Solid Edge part; units mm, degrees
sketch "Sketch1" plane through (0, 0, 0) normal (0, 0, 1) x (1, 0, 0)
  circle A0 centre (10, 5) radius 2.5
  circle A1 centre (10, -5) radius 2.5
  line L0 (-25, -17.5) -> (25, -17.5)
  line L1 (25, -17.5) -> (25, 17.5)
  line L2 (25, 17.5) -> (-25, 17.5)
  line L3 (-25, 17.5) -> (-25, -17.5)
extrude "Protrusion1" add sketch "Sketch1" along normal mid plane 30
sketch "Sketch2" plane through (-25, 0, 0) normal (-1, 0, 0) x (0, -1, 0)
  circle A0 centre (0, 0) radius 10
  circle A1 centre (0, 0) radius 12.5
extrude "ExtrudedProtrusion_2" add sketch "Sketch2" along normal mid plane 50
sketch "Sketch3" plane through (0, 0, 0) normal (0, 0, 1) x (1, 0, 0)
  circle A0 centre (-43, 0) radius 2.25
  circle A1 centre (-33, 0) radius 2.25
extrude "ExtrudedCutout_1" cut sketch "Sketch3" along normal mid plane 87.851
properties material "PVC"
Here's how the part is built. I have some questions about the finished solid (model axes, mm). A direction names the side the tool comes from. Round coordinates to 2 decimals unless told otherwise and drop trailing zeros. Loops run counter-clockwise (first coordinate to the right, second up) from the corner with the lowest first, then second, coordinate; pieces in that order, holes last.
1. If we section it at D-D on x = -33: Write out the boundary of the cut face in (y, z), plus the area to 3 significant figures.
Answer list:
outline: (-2.25, -12.3) - (-2.25, -9.74) arc R10 cw to (-2.25, 9.74) - (-2.25, 12.3) arc R12.5 ccw to start; (2.25, -12.3) arc R12.5 ccw to (2.25, 12.3) - (2.25, 9.74) arc R10 cw to (2.25, -9.74) - close
area: 154 mm2
2. If we section it at C-C on z = 7.5: Write out the boundary of the cut face in (x, y).
Answer list:
outline: (-50, -10) - (-25, -10) - (-25, -17.5) - (25, -17.5) - (25, 17.5) - (-25, 17.5) - (-25, 10) - (-50, 10) - (-50, 6.61) - (-25, 6.61) - (-25, -6.61) - (-50, -6.61) - close; hole circle Ø5 at (10, -5); hole circle Ø5 at (10, 5)
3. If we section it at B-B on y = 0: Write out the boundary of the cut face in (x, z).
Answer list:
outline: (-50, -12.5) - (-45.25, -12.5) - (-45.25, -10) - (-50, -10) - close; (-50, 10) - (-45.25, 10) - (-45.25, 12.5) - (-50, 12.5) - close; (-40.75, -12.5) - (-35.25, -12.5) - (-35.25, -10) - (-40.75, -10) - close; (-40.75, 10) - (-35.25, 10) - (-35.25, 12.5) - (-40.75, 12.5) - close; (-30.75, -12.5) - (-25, -12.5) - (-25, -15) - (25, -15) - (25, 15) - (-25, 15) - (-25, 12.5) - (-30.75, 12.5) - (-30.75, 10) - (-25, 10) - (-25, -10) - (-30.75, -10) - close
4. For P1, Ø7, axis at x = -33, y = 0, coming from the -Z side; P2, Ø2, axis at x = -33.5, y = -3, coming from the -Z side, each with a flat end and sliding along its axis, tell me the tip position at first contact or that it passes through.
Answer list:
P1: stops at z = -12.5
P2: stops at z = -12.33
5. Which directions (+Z, -Z, +X, -X, +Y, -Y) give clear straight access to the entire face, cutting with the end or side of a thin tool? Please do faces 5 (the face through (-37.325, -4.614, 8.872)), 6 (the face through (9.67, 2.52, -0.21)).
Answer list:
face 5: -X
face 6: +Z, -Z
6. If we section it at A-A on x = 10: Write out the boundary of the cut face in (y, z), plus the area to 3 significant figures.
Answer list:
outline: (-17.5, -15) - (-7.5, -15) - (-7.5, 15) - (-17.5, 15) - close; (-2.5, -15) - (2.5, -15) - (2.5, 15) - (-2.5, 15) - close; (7.5, -15) - (17.5, -15) - (17.5, 15) - (7.5, 15) - close
area: 750 mm2
7. If I drill on line 1 along Y through (x, z) = (10, -4.5); line 2 along X through (y, z) = (0, -10.4); line 3 along Y through (x, z) = (11, 3), over which ranges is the centre line in solid material (lowest first)?
Answer list:
line 1: y = -17.5 to -7.5, -2.5 to 2.5, 7.5 to 17.5
line 2: x = -50 to -45.25, -40.75 to -35.25, -30.75 to 25
line 3: y = -17.5 to -7.29, -2.71 to 2.71, 7.29 to 17.5
8. We'd pull the mould along Y, two halves only. Please class faces 1 (the face through (-25, 0, 0)), 2 (the face through (0, 0, -15)), 3 (the face through (0, -17.5, 0)), 4 (the face through (9.67, -7.48, -0.21)): +Y half, -Y half, draft (parallel to the pull), parting line (faces both ways), or undercut.
Answer list:
face 1: undercut
face 2: draft
face 3: -Y half
face 4: undercut
